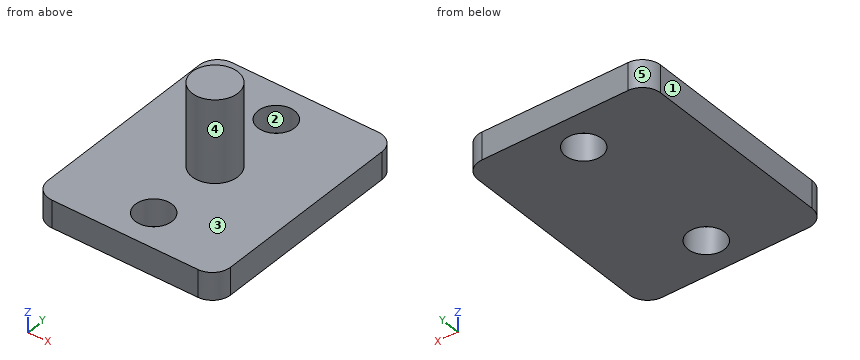
```python
from build123d import *

# Parameters (mm, degrees)
ESQUISSE1_W        = 20
ESQUISSE1_H        = 25
ESQUISSE1_R        = 2
BOSS_EXTRU_1_DEPTH = 3
CONG_1_R           = 2
ESQUISSE2_R        = 2.5
BOSS_EXTRU_3_DEPTH = 9


with BuildPart() as part:
    # Esquisse1 → Boss.-Extru.1 (new body)
    with BuildSketch(Plane.XY):
        Rectangle(ESQUISSE1_W, ESQUISSE1_H)
        with Locations((0, 8.5)):
            Circle(ESQUISSE1_R, mode=Mode.SUBTRACT)
        with Locations(Location((0, -8.5, 0), (0, 0, 180))):
            Circle(ESQUISSE1_R, mode=Mode.SUBTRACT)
    extrude(amount=BOSS_EXTRU_1_DEPTH)

    # Congé1
    cong_1_edges = [part.edges().sort_by_distance(p)[0] for p in [
        (-10, 12.5, 1.5),
        (10, 12.5, 1.5),
        (10, -12.5, 1.5),
        (-10, -12.5, 1.5),
    ]]
    fillet(cong_1_edges, radius=CONG_1_R)

    # Esquisse2 → Boss.-Extru.3 (add)
    with BuildSketch(Plane.XY.offset(3)):
        Circle(ESQUISSE2_R)
    extrude(amount=BOSS_EXTRU_3_DEPTH)


solid = part.part
```
Read the model definition and answer for the solid it produces. Units are mm, in the model's axes. Face numbers are marked on the shaded views. A direction names the side the tool comes from. Round coordinates to 2 decimals unless told otherwise and drop trailing zeros. Loops run counter-clockwise (first coordinate to the right, second up) from the corner with the lowest first, then second, coordinate; pieces in that order, holes last. Notation, with made-up numbers: (79.25, 32) -> (92.25, 32) arc R19 ccw to (92.25, 62) -> close; hole circle Ø11 at (2, 75.5). An arc over 180 degrees is marked (long way). One line per item, written item: value.
1) A cutting plane is placed at B-B (y = -8.5). Determine the outline of the cut face in (x, z).
Answer list:
outline: (-10, 0) -> (-2, 0) -> (-2, 3) -> (-10, 3) -> close; (2, 0) -> (10, 0) -> (10, 3) -> (2, 3) -> close
2) A cutting plane is placed at A-A (x = 0). Determine the outline of the cut face in (y, z), and give its area (3 significant figures).
Answer list:
outline: (-12.5, 0) -> (-10.5, 0) -> (-10.5, 3) -> (-12.5, 3) -> close; (-6.5, 0) -> (6.5, 0) -> (6.5, 3) -> (2.5, 3) -> (2.5, 12) -> (-2.5, 12) -> (-2.5, 3) -> (-6.5, 3) -> close; (10.5, 0) -> (12.5, 0) -> (12.5, 3) -> (10.5, 3) -> close
area: 96.0 mm²
3) A cutting plane is placed at C-C (y = -0.75). Determine the outline of the cut face in (x, z), and give its area (3 significant figures).
Answer list:
outline: (-10, 0) -> (10, 0) -> (10, 3) -> (2.38, 3) -> (2.38, 12) -> (-2.38, 12) -> (-2.38, 3) -> (-10, 3) -> close
area: 103 mm²
4) The mould has two halves that part along X. Classify the marked faces 1, 2 and 3: pulls with the +X half, pulls with the -X half, needs draft (parallel to the pull), parting line crosses it, or undercut.
Answer list:
face 1: pulls with the -X half
face 2: undercut
face 3: needs draft
5) For the marked faces 4 and 5, determine the directions among +Z, -Z, +X, -X, +Y, -Y from which every point of the face is accessible in a straight line to the end or side of a thin tool.
Answer list:
face 4: +Z
face 5: +Z, -Z, -X, +Y
6) A flat-ended cylindrical pin translates along its axis: P1, Ø4.5, axis at x = 0, y = -8.5, coming from the +Z side. Find the tip coordinate at first contact, or state that the pin passes through.
Answer list:
P1: stops at z = 3
7) Consider L1, parallel to Y at x = 0, z = 1.9; L2, parallel to Z at x = -5.5, y = -11; L3, parallel to Y at x = 1.5, z = 11.5. Determine where each line is inside the solid, lowest interval first. Write a range as [from, to].
Answer list:
L1: y = [-12.5, -10.5], [-6.5, 6.5], [10.5, 12.5]
L2: z = [0, 3]
L3: y = [-2, 2]
8) A cutting plane is placed at D-D (x = 6.25). Determine the outline of the cut face in (y, z).
Answer list:
outline: (-12.5, 0) -> (12.5, 0) -> (12.5, 3) -> (-12.5, 3) -> close
